from build123d import *

# Parameters (mm, degrees)
EXTRUDE_1_DEPTH = 1200
FILLET_1_R      = 1


with BuildPart() as part:
    # Sketch 1 → Extrude 1 (new body)
    with BuildSketch(Plane(origin=(0, 0, 0), x_dir=(1, 0, 0), z_dir=(0, 1, 0))):
        with BuildLine():
            Line((2.337006084, 17.550433348), (-7.851124943, 17.550433348))
            Line((-7.851124943, 17.550433348), (-7.851124943, 18.550433348))
            Line((-7.851124943, 18.550433348), (5.337006084, 18.550433348))
            ThreePointArc((5.337006084, 18.550433348), (9.933200162, 16.646627425), (11.837006084, 12.050433348))
            Line((11.837006084, 12.050433348), (11.837006084, -5.16889475))
            Line((11.837006084, -5.16889475), (10.837006084, -5.16889475))
            Line((10.837006084, -5.16889475), (10.837006084, 9.050433348))
            ThreePointArc((10.837006084, 9.050433348), (8.861760963, 12.039998533), (5.337006084, 11.395641227))
            Line((5.337006084, 11.395641227), (5.337006084, -5.16889475))
            Line((5.337006084, -5.16889475), (4.337006084, -5.16889475))
            Line((4.337006084, -5.16889475), (4.337006084, 11.050433348))
            Line((4.337006084, 11.050433348), (-7.851124943, 11.050433348))
            Line((-7.851124943, 11.050433348), (-7.851124943, 12.050433348))
            Line((-7.851124943, 12.050433348), (4.682213964, 12.050433348))
            ThreePointArc((4.682213964, 12.050433348), (5.32657127, 15.575188226), (2.337006084, 17.550433348))
        make_face()
    extrude(amount=EXTRUDE_1_DEPTH)

    # Fillet 1
    fillet_1_edges = [part.edges().sort_by_distance(p)[0] for p in [
        (5.337006084, 600, -11.395641227),
        (4.337006084, 600, -11.050433348),
        (4.682213964, 600, -12.050433348),
    ]]
    fillet(fillet_1_edges, radius=FILLET_1_R)


solid = part.part
Input: part model. Units: mm. Frame: model coordinates. Give positions to 0.01 mm unless a question says otherwise; leave off trailing zeros. Order: outer loops, then holes, each group sorted by start corner. A loop starts at its lowest first (then second) coordinate and runs counter-clockwise, first axis right, second up.
Q1. Section A-A on z = -1.25. Output: boundary loops of the cut face in (x, y).
Checked values:
outline: (4.34, 0) - (5.34, 0) - (5.34, 1200) - (4.34, 1200) - close; (10.84, 0) - (11.84, 0) - (11.84, 1200) - (10.84, 1200) - close
Q2. Section B-B on x = -1.5. Output: boundary loops of the cut face in (y, z), and give its area (3 significant figures).
Checked values:
outline: (0, -18.55) - (1200, -18.55) - (1200, -17.55) - (0, -17.55) - close; (0, -12.05) - (1200, -12.05) - (1200, -11.05) - (0, -11.05) - close
area: 2,400 mm2
Q3. Ray query, probe 1 along Z at (x, y) = (-6, 289); probe 2 along X at (y, z) = (1041.5, -1.25). Return the intervals inside material, ascending.
Checked values:
probe 1: z = -18.55 to -17.55, -12.05 to -11.05
probe 2: x = 4.34 to 5.34, 10.84 to 11.84
Q4. Contact query for flat-ended pins moving along their axis: pin 1 Ø4.5 at (y, z) = (504, 1) entering from -X; pin 2 Ø5 at (x, y) = (-1, 741) entering from +Z; pin 3 Ø11.5 at (y, z) = (649.5, -5) entering from -X; pin 4 Ø10 at (x, z) = (-2, -9) entering from -Y. Output: stop coordinate, or through.
Checked values:
pin 1: stops at x = 4.34
pin 2: stops at z = -11.05
pin 3: stops at x = 4.05
pin 4: stops at y = 0
Q5. Section C-C on y = 690. Output: boundary loops of the cut face in (x, z).
Checked values:
outline: (-7.85, -18.55) - (5.34, -18.55) arc R6.5 ccw to (11.84, -12.05) - (11.84, 5.17) - (10.84, 5.17) - (10.84, -9.05) arc R3.25 cw to (5.78, -11.75) arc R1 cw to (5.34, -10.92) - (5.34, 5.17) - (4.34, 5.17) - (4.34, -10.05) arc R1 cw to (3.34, -11.05) - (-7.85, -11.05) - (-7.85, -12.05) - (4.21, -12.05) arc R1 cw to (5.04, -12.49) arc R3.25 cw to (2.34, -17.55) - (-7.85, -17.55) - close
